Work out the finished part from the listing and answer in its coordinate system (mm). A direction names the side the tool comes from. Round coordinates to 2 decimals unless told otherwise and drop trailing zeros. Write each loop counter-clockwise with the first axis right and the second up, starting at its lowest first coordinate (ties: lowest second). Pieces come first, ordered by that corner, then holes.
from build123d import *

# Parameters (mm, degrees)
F0_R     = 203.2
F1_DEPTH = 1016
F2_R     = 228.6
F3_DEPTH = 812.8
F5_W     = 533.122748
F5_H     = 457.2
F6_DEPTH = 812.801
F5_W_2   = 649.697065
F7_DEPTH = 812.801


with BuildPart() as f1:
    # F0 (on Front) → F1 (new body)
    with BuildSketch(Plane.XZ):
        with BuildLine():
            Line((14.697065, 56.260465), (929.097065, 56.260465))
            Line((929.097065, 56.260465), (929.097065, 868.794625))
            Line((929.097065, 868.794625), (0, 868.794625))
            ThreePointArc((0, 868.794625), (-406.333535, 455.04489), (14.697065, 56.260465))
        make_face()
        with Locations((0, 462.394625)):
            Circle(F0_R, mode=Mode.SUBTRACT)
    extrude(amount=F1_DEPTH)

    # F2 (on face) → F3 (join)
    with BuildSketch(Plane.YZ.offset(929.097065)):
        with Locations((-508, 462.394625)):
            Circle(F2_R)
    extrude(amount=F3_DEPTH)

    # F5 (on face) → F6 (cut, through all)
    with BuildSketch(Plane.XY.offset(868.794625)):
        with Locations((-266.561374, -508)):
            Rectangle(F5_W, F5_H)
    extrude(amount=-F6_DEPTH, mode=Mode.SUBTRACT)

    # F5 (on face) → F7 (cut, through all)
    with BuildSketch(Plane.XY.offset(868.794625)):
        with Locations((324.848532, -508)):
            Rectangle(F5_W_2, F5_H)
        with Locations((-266.561374, -508)):
            Rectangle(F5_W, F5_H)
    extrude(amount=-F7_DEPTH, mode=Mode.SUBTRACT)


solid = f1.part
Q1. Given pin 1 (2 mm diameter, centred on x = 93.5, y = -210, fed in from -Z); pin 2 (2 mm diameter, centred on y = -583, z = 701.5, fed in from -X); pin 3 (1.5 mm diameter, centred on x = 954.5, z = 578.5, fed in from -Y), each flat-ended and moving along its own axis, determine where each tip first touches the part or whether it passes through.
Q2. Find the intervals of material crossed by L1, parallel to Z at x = 0, y = -132; L2, parallel to Y at x = 570, z = 441; L3, parallel to X at y = -629, z = 558, in increasing order.
Q3. Find section B-B (z = 489.5). Determine the outline of the cut face in (x, y), plus the area to 3 significant figures.
Q4. Find section A-A (y = -508). Determine the outline of the cut face in (x, z), plus the area to 3 significant figures.
Q5. A tool of negligible diameter and unlimited length cuts with its end or side. For faces 4 (the face through (929.097, -275, 457)), 5 (the face through (232, -736.6, 468)), 6 (the face through (-44.05, -874.344, 264.027)), from which of +Z, -Z, +X, -X, +Y, -Y can it reach the whole face along a straight path? Write none if from no direction.
Q6. The mould has two halves that part along Z. Classify faces 1 (the face through (246, -279.4, 468)), 2 (the face through (1329.807, -289.956, 531.06)), 3 (the face through (-44.05, -137.744, 264.027)): +Z half, -Z half, draft (parallel to the pull), parting line (faces both ways), or undercut.
Q7. Find section D-D (y = -829). Determine the outline of the cut face in (x, z).
Q8. Find section C-C (z = 148.5). Determine the outline of the cut face in (x, y), plus the area to 3 significant figures.
Report:
1. pin 1: stops at z = 56.26
1. pin 2: stops at x = 649.7
1. pin 3: stops at y = -705.36
2. L1: z = 55.99 to 259.19, 665.59 to 868.79
2. L2: y = -1016 to -736.6, -279.4 to 0
2. L3: x = 649.7 to 1741.9
3. outline: (-405.5, -1016) - (-201.38, -1016) - (-201.38, -736.6) - (-405.5, -736.6) - close; (-405.5, -279.4) - (-201.38, -279.4) - (-201.38, 0) - (-405.5, 0) - close; (201.38, -1016) - (929.1, -1016) - (929.1, -734.99) - (1741.9, -734.99) - (1741.9, -281.01) - (929.1, -281.01) - (929.1, 0) - (201.38, 0) - (201.38, -279.4) - (649.7, -279.4) - (649.7, -736.6) - (201.38, -736.6) - close
3. area: 1,020,000 mm2
4. outline: (649.7, 56.26) - (929.1, 56.26) - (929.1, 233.79) - (1741.9, 233.79) - (1741.9, 690.99) - (929.1, 690.99) - (929.1, 868.79) - (649.7, 868.79) - close
4. area: 599,000 mm2
5. face 4: +X
5. face 5: +Z, -Z, -X
5. face 6: +Y, -Y
6. face 1: draft
6. face 2: parting line
6. face 3: undercut
7. outline: (0, 868.79) arc R406.4 ccw (long way) to (14.7, 56.26) - (929.1, 56.26) - (929.1, 868.79) - close; hole circle Ø406.4 at (0, 462.39)
8. outline: (-258.13, -1016) - (929.1, -1016) - (929.1, 0) - (-258.13, 0) - (-258.13, -279.4) - (649.7, -279.4) - (649.7, -736.6) - (-258.13, -736.6) - close
8. area: 791,000 mm2
